from build123d import *

# Parameters (mm, degrees)
SKETCH_W        = 29.5
SKETCH_H        = 40
SKETCH_R        = 1.75
PAD_DEPTH       = 24
SKETCH001_W     = 25.5
SKETCH001_H     = 36
POCKET_DEPTH    = 20
POCKET001_DEPTH = 29.501
SKETCH003_R     = 6.5
POCKET002_DEPTH = 5


with BuildPart() as part:
    # Sketch → Pad (new body)
    with BuildSketch(Plane.XY):
        with Locations((0, 10)):
            Rectangle(SKETCH_W, SKETCH_H)
        with Locations((-8.25, 14)):
            Circle(SKETCH_R, mode=Mode.SUBTRACT)
        with Locations((0, 14)):
            Circle(SKETCH_R, mode=Mode.SUBTRACT)
        with Locations((8.25, 14)):
            Circle(SKETCH_R, mode=Mode.SUBTRACT)
    extrude(amount=PAD_DEPTH)

    # Sketch001 (on Face9 of Pad) → Pocket (cut)
    with BuildSketch(Plane.XY.offset(24)):
        with Locations((0, 12)):
            Rectangle(SKETCH001_W, SKETCH001_H)
    extrude(amount=-POCKET_DEPTH, mode=Mode.SUBTRACT)

    # Sketch002 (on Face8 of Pocket) → Pocket001 (cut, through all)
    with BuildSketch(Plane(origin=(-14.75, 0, 0), x_dir=(0, -1, 0), z_dir=(-1, 0, 0))):
        Polygon((-30, 24), (6, 24), (-30, 4), align=None)
    extrude(amount=-POCKET001_DEPTH, mode=Mode.SUBTRACT)

    # Sketch003 (on Face15 of Pocket001) → Pocket002 (cut)
    with BuildSketch(Plane(origin=(0, -6, 0), x_dir=(-1, 0, 0), z_dir=(0, 1, 0))):
        with Locations((0.044684, 14)):
            Circle(SKETCH003_R)
    extrude(amount=-POCKET002_DEPTH, mode=Mode.SUBTRACT)


solid = part.part
Verification items for the finished model (mm, model axes). A direction names the side the tool comes from. Round coordinates to 2 decimals unless told otherwise and drop trailing zeros. Loops run counter-clockwise (first coordinate to the right, second up) from the corner with the lowest first, then second, coordinate; pieces in that order, holes last. Notation, with made-up numbers: (11.5, 19) - (45.5, 19) arc R25 ccw to (45.5, 54) - close; hole circle Ø1 at (-38.5, 6.25). An arc over 180 degrees is marked (long way). Use a Markdown table: item, result. Add a question column.
1. Release check for a two-part mould opening along X. For faces 3 (the face through (0, 10, 0)), 4 (the face through (-14.75, 5, 9)), 5 (the face through (12.75, 4, 10)) record: released by +X, released by -X, zero draft, split by the parting line, or undercut.
2. Section check D-D, the plane z = 6.5. Record the boundary of the cut face in (x, y), plus the area to 3 significant figures.
3. Section check A-A, the plane x = 8.25. Record the boundary of the cut face in (y, z), plus the area to 3 significant figures.
4. Gauge pin test, flat ends, axial feed: pin 1 (2 mm diameter, centred on x = -11, y = -5.5, fed in from +Z); pin 2 (2 mm diameter, centred on x = -9, y = 10.5, fed in from +Z). Record the tip position at first contact, or that the pin passes through.
5. Section check C-C, the plane y = 14. Record the boundary of the cut face in (x, z).
6. Section check B-B, the plane z = 14. Record the boundary of the cut face in (x, y), plus the area to 3 significant figures.
7. Access from +Z, -Z, +X, -X, +Y, -Y to the whole of each face (thin tool, end or side, straight path). Record for faces 1 (the face through (0, -6, 21)), 2 (the face through (-14, 12, 14)).
8. Thickness scan on probe 1 along X at (y, z) = (14, 2.05); probe 2 along Y at (x, z) = (8.25, 2.7); probe 3 along X at (y, z) = (7.5, 7.25). Record the ranges inside material, lowest first. Write a range as [from, to].
Checks:
| question | item | result |
|---|---|---|
| 1 | face 3 | zero draft |
| 1 | face 4 | released by -X |
| 1 | face 5 | undercut |
| 2 | outline | (-14.75, -10) - (14.75, -10) - (14.75, 25.5) - (12.75, 25.5) - (12.75, -6) - (-12.75, -6) - (-12.75, 25.5) - (-14.75, 25.5) - close |
| 2 | area | 244 mm^2 |
| 3 | outline | (-10, 0) - (12.25, 0) - (12.25, 4) - (-6, 4) - (-6, 24) - (-10, 24) - close; (15.75, 0) - (30, 0) - (30, 4) - (15.75, 4) - close |
| 3 | area | 226 mm^2 |
| 4 | pin 1 | stops at z = 24 |
| 4 | pin 2 | stops at z = 4 |
| 5 | outline | (-14.75, 0) - (-10, 0) - (-10, 4) - (-12.75, 4) - (-12.75, 12.89) - (-14.75, 12.89) - close; (-6.5, 0) - (-1.75, 0) - (-1.75, 4) - (-6.5, 4) - close; (1.75, 0) - (6.5, 0) - (6.5, 4) - (1.75, 4) - close; (10, 0) - (14.75, 0) - (14.75, 12.89) - (12.75, 12.89) - (12.75, 4) - (10, 4) - close |
| 6 | outline | (-14.75, -10) - (-6.54, -10) - (-6.54, -6) - (-12.75, -6) - (-12.75, 12) - (-14.75, 12) - close; (6.46, -10) - (14.75, -10) - (14.75, 12) - (12.75, 12) - (12.75, -6) - (6.46, -6) - close |
| 6 | area | 138 mm^2 |
| 7 | face 1 | +Z, +Y |
| 7 | face 2 | +Z, +X, -X, +Y |
| 8 | probe 1 | x = [-14.75, -10], [-6.5, -1.75], [1.75, 6.5], [10, 14.75] |
| 8 | probe 2 | y = [-10, 12.25], [15.75, 30] |
| 8 | probe 3 | x = [-14.75, -12.75], [12.75, 14.75] |
